Model file for the job. Use its own axes, mm. Give positions to 0.01 mm unless a question says otherwise; leave off trailing zeros. Loops run counter-clockwise (first coordinate to the right, second up) from the corner with the lowest first, then second, coordinate; pieces in that order, holes last. Notation, with made-up numbers: M 43.5,-11.75 L 68.5,-11.75 A6 cw 68.5,-0.75 Z; hole C 79.25,20.5 d10. An arc over 180 degrees is marked long. Answer in a Markdown table with one row per item.
```python
from build123d import *

# Parameters (mm, degrees)
SKETCH002_W         = 6
SKETCH002_H         = 48
PAD001_DEPTH        = 6
PAD001_DEPTH_BACK   = 30
PAD002_DEPTH        = 3
HOLE004_D           = 4.5
HOLE004_DEPTH       = 25
HOLE004_CSINK_D     = 6.1
HOLE004_CSINK_ANGLE = 90


with BuildPart() as part:
    # Sketch002 (on Face1 of Binder001) → Pad001 (new body, two sides)
    with BuildSketch(Plane.XY) as pad001_sk:
        with Locations((-24, 0)):
            Rectangle(SKETCH002_W, SKETCH002_H)
    extrude(amount=PAD001_DEPTH)
    extrude(pad001_sk.sketch, amount=-PAD001_DEPTH_BACK)

    # Sketch003 (on Face3 of Pad001) → Pad002 (join)
    with BuildSketch(Plane.XZ.offset(24)):
        Polygon((-21, 0), (-21, -7), (-17, 0), align=None)
    pad002 = extrude(amount=-PAD002_DEPTH)

    # Mirrored: Pad002 across XZ
    add(pad002.mirror(Plane.XZ))

    # Hole004
    with Locations(Plane(origin=(-21, -191, 0), x_dir=(0, -1, 0), z_dir=(1, 0, 0))):
        with Locations((-189.999737, 25.501831), (-182.5, 12.5)):
            CounterSinkHole(HOLE004_D / 2, HOLE004_CSINK_D / 2, depth=HOLE004_DEPTH, counter_sink_angle=HOLE004_CSINK_ANGLE)


solid = part.part
```
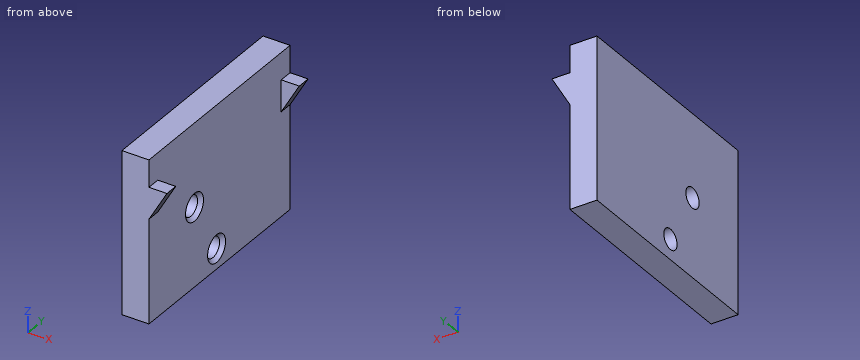
(1) Saw through at B-B, the plane y = -8.5. Give the cut face in (x, z).
Established:
| item | result |
|---|---|
| outline | M -27,-30 L -21,-30 L -21,-15.55 L -21.8,-14.75 L -27,-14.75 Z; M -27,-10.25 L -21.8,-10.25 L -21,-9.45 L -21,6 L -27,6 Z |
(2) Wall check: L1, parallel to Y at x = -25.1, z = -12.5; L2, parallel to Z at x = -23, y = -8.5; L3, parallel to X at y = 10.5, z = -12. Give the ranges that are in metal, low to high.
Established:
| item | result |
|---|---|
| L1 | y = -24 to -10.75, -6.25 to 24 |
| L2 | z = -30 to -14.75, -10.25 to 6 |
| L3 | x = -27 to -21 |
(3) Saw through at D-D, the plane z = -6.5. Give the cut face in (x, y).
Established:
| item | result |
|---|---|
| outline | M -27,-24 L -20.71,-24 L -20.71,-21 L -21,-21 L -21,21 L -20.71,21 L -20.71,24 L -27,24 Z |
(4) Saw through at C-C, the plane x = -19.5. Give the cut face in (y, z) (3 decimals), and give its area (4 significant figures).
Established:
| item | result |
|---|---|
| outline | M -24,-4.375 L -21,-4.375 L -21,0 L -24,0 Z; M 21,-4.375 L 24,-4.375 L 24,0 L 21,0 Z |
| area | 26.25 mm2 |
(5) Saw through at A-A, the plane z = -12.5. Give the cut face in (x, y), and give its area (3 significant figures).
Established:
| item | result |
|---|---|
| outline | M -27,-24 L -21,-24 L -21,-11.55 L -21.8,-10.75 L -27,-10.75 Z; M -27,-6.25 L -21.8,-6.25 L -21,-5.45 L -21,24 L -27,24 Z |
| area | 260 mm2 |
(6) Flat gauge pins, fed straight in: P1, Ø0.9, axis at x = -20, y = 23, coming from the +Z side; P2, Ø3, axis at y = -14.5, z = -22.5, coming from the +X side; P3, Ø3.5, axis at y = -8.5, z = -12.5, coming from the +X side. Where does each tip first touch, or does it go through?
Established:
| item | result |
|---|---|
| P1 | stops at z = 0 |
| P2 | stops at x = -21 |
| P3 | passes through |
